Autodesk Inventor part; units mm, degrees
ref_plane "YZ Plane" through (0, 0, 0) normal (1, 0, 0) x (0, 1, 0)
ref_plane "XZ Plane" through (0, 0, 0) normal (0, 1, 0) x (-1, 0, 0)
ref_plane "XY Plane" through (0, 0, 0) normal (0, 0, 1) x (1, 0, 0)
sketch "Sketch1" plane through (0, 0, 0) normal (0, 0, 1) x (1, 0, 0)
  line L0 (-40, 55.2261) -> (40, 55.2261)
  line L1 (40, 55.2261) -> (40, -24.3415)
  line L2 (40, -24.3415) -> (-40, -24.3415)
  line L3 (-40, -24.3415) -> (-40, 55.2261)
  point P0 (0, 0)
  dimension "d8" = 24.3415
extrude "Extrusion1" add sketch "Sketch1" against normal blind 2
sketch "Sketch2" plane through (0, 0, 0) normal (0, 0, 1) x (1, 0, 0)
  line L0 (-40, 55.2261) -> (40, 55.2261)
  line L1 (-40, 55.2261) -> (39.9042, 55.2261) construction
  line L2 (39.9042, 55.2261) -> (39.9042, -24.6781) construction
  line L3 (39.9042, -24.6781) -> (-40, -24.6781) construction
  line L4 (-40, -24.6781) -> (-40, 55.2261) construction
  point P0 (0, 0)
sketch "Sketch3" plane through (0, 0, 0) normal (0, 0, 1) x (1, 0, 0)
  line L0 (40, -24.3415) -> (-40, -24.3415)
  line L1 (-5, -24.3415) -> (5, -24.3415)
  line L2 (5, -24.3415) -> (5, -94.3415)
  line L3 (5, -94.3415) -> (-5, -94.3415)
  line L4 (-5, -94.3415) -> (-5, -24.3415)
  line L5 (-15, -94.3415) -> (15, -94.3415)
  line L6 (15, -94.3415) -> (15, -104.3415)
  line L7 (15, -104.3415) -> (-15, -104.3415)
  line L8 (-15, -104.3415) -> (-15, -94.3415)
  point P0 (0, 0)
  dimension "d12" = 10
  dimension "d13" = 70
  dimension "d14" = 5
  dimension "d15" = 30
  dimension "d16" = 10
extrude "Extrusion2" add sketch "Sketch3" along normal mid plane 10 contours L5 L6 L7 L8 L3
sketch "Sketch4" plane through (0, 0, 5) normal (0, 0, 1) x (1, 0, 0)
  point P0 (0, 0)
sketch "Sketch7" plane through (0, 0, -2) normal (0, 0, -1) x (-1, 0, 0)
  line L0 (-40, -24.3415) -> (40, -24.3415)
  line L1 (-15, -94.3415) -> (15, -94.3415)
  line L2 (-4.9075, -24.3415) -> (5.0925, -24.3415)
  line L3 (5.0925, -24.3415) -> (5.0925, -94.3415)
  line L4 (5.0925, -94.3415) -> (-4.9075, -94.3415)
  line L5 (-4.9075, -94.3415) -> (-4.9075, -24.3415)
  point P0 (0, 0)
  dimension "d21" = 10
extrude "Extrusion3" add sketch "Sketch7" against normal blind 2
properties part number "parkinglot"
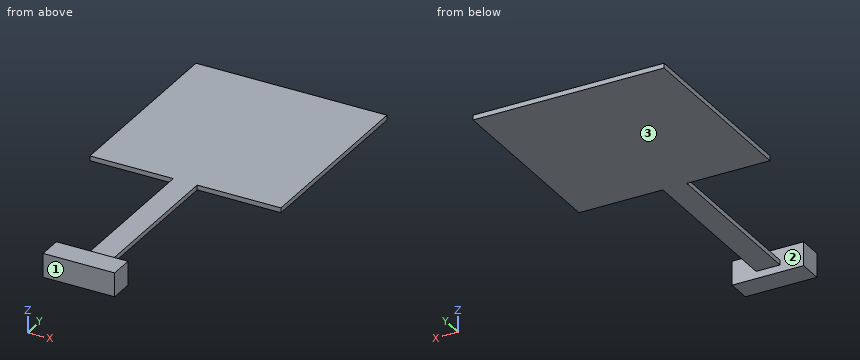
Check sheet for the modelled part. Datum: model origin and axes. Units: mm. Face numbers are marked on the shaded views. Round coordinates to 2 decimals unless told otherwise and drop trailing zeros. Loops run counter-clockwise (first coordinate to the right, second up) from the corner with the lowest first, then second, coordinate; pieces in that order, holes last.
1. Sectioned sample at D-D on z = 2.25. Record the boundary of the cut face in (x, y), and give its area (3 significant figures).
2. Gauge pin test, flat ends, axial feed: pin 1 Ø1.5 at (x, z) = (17.5, -1) entering from -Y; pin 2 Ø3 at (y, z) = (-97.5, 0.5) entering from -X; pin 3 Ø6 at (y, z) = (3.5, 4) entering from -X; pin 4 Ø2 at (y, z) = (-51.5, -1.5) entering from -X. Record the tip position at first contact, or that the pin passes through.
3. Sectioned sample at A-A on x = -8. Record the boundary of the cut face in (y, z), and give its area (3 significant figures).
4. Sectioned sample at C-C on y = 27.5. Record the boundary of the cut face in (x, z).
5. Mould release check, pull along Y, two halves, no side actions. Record for the marked faces 1, 2 and 3: released by +Y, released by -Y, zero draft, split by the parting line, or undercut.
6. Scan lines: probe 1 along Z at (x, y) = (-21.5, 14.5); probe 2 along Y at (x, z) = (14, 1.75); probe 3 along Y at (x, z) = (19.5, -1). Record each from-to range of solid material in increasing order.
7. Sectioned sample at B-B on x = 0. Record the boundary of the cut face in (y, z), and give its area (3 significant figures).
Recorded:
1. outline: (-15, -104.34) - (15, -104.34) - (15, -94.34) - (-15, -94.34) - close
1. area: 300 mm2
2. pin 1: stops at y = -24.34
2. pin 2: stops at x = -15
2. pin 3: passes through
2. pin 4: stops at x = -5.09
3. outline: (-104.34, -5) - (-94.34, -5) - (-94.34, 5) - (-104.34, 5) - close; (-24.34, -2) - (55.23, -2) - (55.23, 0) - (-24.34, 0) - close
3. area: 259 mm2
4. outline: (-40, -2) - (40, -2) - (40, 0) - (-40, 0) - close
5. face 1: released by -Y
5. face 2: undercut
5. face 3: zero draft
6. probe 1: z = -2 to 0
6. probe 2: y = -104.34 to -94.34
6. probe 3: y = -24.34 to 55.23
7. outline: (-104.34, -5) - (-94.34, -5) - (-94.34, -2) - (55.23, -2) - (55.23, 0) - (-94.34, 0) - (-94.34, 5) - (-104.34, 5) - close
7. area: 399 mm2
